For this review, take the finished solid that the model builds, in its own axes (mm). A direction names the side the tool comes from. Give positions to 0.01 mm unless a question says otherwise; leave off trailing zeros. Loops run counter-clockwise (first coordinate to the right, second up) from the corner with the lowest first, then second, coordinate; pieces in that order, holes last.
```python
from build123d import *

# Parameters (mm, degrees)
SKETCH_1_R          = 15
EXTRUDE_1_DEPTH     = 2
SKETCH_2_R          = 5
SKETCH_2_R_2        = 4
EXTRUDE_2_DEPTH     = 12
CUT_EXTRUDE_START   = -12
SKETCH_3_R          = 4
CUT_EXTRUDE_1_DEPTH = 12
SKETCH_4_R          = 1.6
CUT_EXTRUDE_2_DEPTH = 12


with BuildPart() as part:
    # 草图1 → 凸台-拉伸1 (new body)
    with BuildSketch(Plane(origin=(0, 0, 0), x_dir=(1, 0, 0), z_dir=(0, 1, 0))):
        with Locations(Location((0, 0, 0), (0, 0, 270))):
            Circle(SKETCH_1_R)
    extrude(amount=EXTRUDE_1_DEPTH)

    # 草图2 → 凸台-拉伸2 (add)
    with BuildSketch(Plane(origin=(0, 2, 0), x_dir=(1, 0, 0), z_dir=(0, 1, 0))):
        with Locations(Location((0, 0, 0), (0, 0, 270))):
            Circle(SKETCH_2_R)
        with Locations(Location((0, 0, 0), (0, 0, 270))):
            Circle(SKETCH_2_R_2, mode=Mode.SUBTRACT)
    extrude(amount=EXTRUDE_2_DEPTH)

    # 草图3 → 切除-拉伸1 (cut)
    with BuildSketch(Plane(origin=(0, 2, 0), x_dir=(1, 0, 0), z_dir=(0, 1, 0)).offset(CUT_EXTRUDE_START)):
        with Locations(Location((0, 0, 0), (0, 0, 270))):
            Circle(SKETCH_3_R)
    extrude(amount=CUT_EXTRUDE_1_DEPTH, mode=Mode.SUBTRACT)

    # 草图4 → 切除-拉伸2 (cut)
    with BuildSketch(Plane(origin=(0, 2, 0), x_dir=(1, 0, 0), z_dir=(0, 1, 0))):
        with Locations(Location((0, 10.5, 0), (0, 0, 270))):
            Circle(SKETCH_4_R)
        with Locations(Location((10.5, 0, 0), (0, 0, 270))):
            Circle(SKETCH_4_R)
        with Locations(Location((0, -10.5, 0), (0, 0, 270))):
            Circle(SKETCH_4_R)
        with Locations(Location((-10.5, 0, 0), (0, 0, 270))):
            Circle(SKETCH_4_R)
    extrude(amount=-CUT_EXTRUDE_2_DEPTH, mode=Mode.SUBTRACT)


solid = part.part
```
Q1. For pin 1 Ø1 at (y, z) = (9, 3) entering from +X; pin 2 Ø3.5 at (x, z) = (0, -10.5) entering from +Y; pin 3 Ø13 at (x, z) = (0, 0) entering from -Y; pin 4 Ø1 at (y, z) = (4.5, -5) entering from +X, all flat-tipped, find the tip position at first contact; note any pin that passes through.
Answers:
pin 1: stops at x = 4.33
pin 2: stops at y = 2
pin 3: stops at y = 0
pin 4: stops at x = 2.18
Q2. Consider section B-B on z = 0. Give the boundary of the cut face in (x, y), plus the area to 3 significant figures.
Answers:
outline: (-15, 0) - (-12.1, 0) - (-12.1, 2) - (-15, 2) - close; (-8.9, 0) - (-4, 0) - (-4, 14) - (-5, 14) - (-5, 2) - (-8.9, 2) - close; (4, 0) - (8.9, 0) - (8.9, 2) - (5, 2) - (5, 14) - (4, 14) - close; (12.1, 0) - (15, 0) - (15, 2) - (12.1, 2) - close
area: 55.2 mm2
Q3. For probe 1 along X at (y, z) = (0.45, 0); probe 2 along Y at (x, z) = (8, -10.75); probe 3 along X at (y, z) = (1.25, -1.75), list the stretches that pass through material, from the lowest coordinate up.
Answers:
probe 1: x = -15 to -12.1, -8.9 to -4, 4 to 8.9, 12.1 to 15
probe 2: y = 0 to 2
probe 3: x = -14.9 to -3.6, 3.6 to 14.9
Q4. Machinability: for faces 1 (the cylindrical face through (-12.06, 1.01, -0.35)), 2 (the cylindrical face through (-4.88, 7.92, -1.08)), which of the approach directions +Z, -Z, +X, -X, +Y, -Y give a long, thin tool a straight path to every point of the face, cutting with its end or side? Answer none if there is none.
Answers:
face 1: +Y, -Y
face 2: +Y
Q5. Consider section C-C on z = 10.5. Give the boundary of the cut face in (x, y), plus the area to 3 significant figures.
Answers:
outline: (-10.71, 0) - (-1.6, 0) - (-1.6, 2) - (-10.71, 2) - close; (1.6, 0) - (10.71, 0) - (10.71, 2) - (1.6, 2) - close
area: 36.4 mm2
Q6. Consider section D-D on x = -10.5. Give the boundary of the cut face in (y, z).
Answers:
outline: (0, -10.71) - (2, -10.71) - (2, -1.6) - (0, -1.6) - close; (0, 1.6) - (2, 1.6) - (2, 10.71) - (0, 10.71) - close
Q7. Mouldability with a two-part tool opening along Z and no side actions: class faces 3 (the cylindrical face through (0.07, 1.01, -12.1)), 4 (the flat face through (4, 2, -4)), 5 (the cylindrical face through (0.66, 0.986, -14.985)) as +Z half, -Z half, draft (parallel to the pull), parting line (faces both ways), or undercut.
Answers:
face 3: undercut
face 4: draft
face 5: parting line
Q8. Consider section A-A on x = 0. Give the boundary of the cut face in (y, z).
Answers:
outline: (0, -15) - (2, -15) - (2, -12.1) - (0, -12.1) - close; (0, -8.9) - (2, -8.9) - (2, -5) - (14, -5) - (14, -4) - (0, -4) - close; (0, 4) - (14, 4) - (14, 5) - (2, 5) - (2, 8.9) - (0, 8.9) - close; (0, 12.1) - (2, 12.1) - (2, 15) - (0, 15) - close
